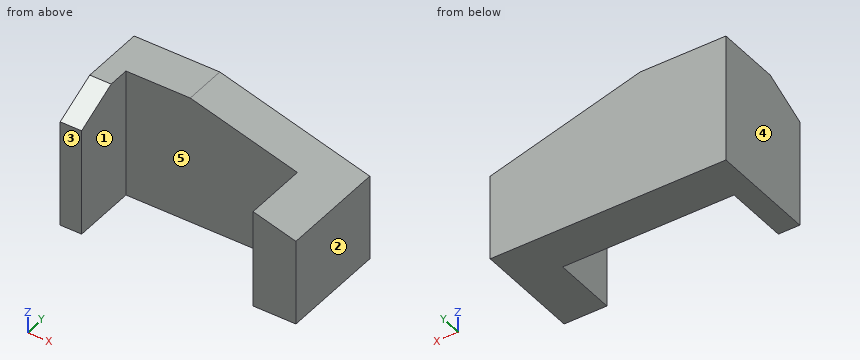
from build123d import *

# Parameters (mm, degrees)
F0_W     = 10
F0_H     = 20
F1_DEPTH = 60
F2_SIZE2 = 20
F2_SIZE  = 70
F3_SIZE2 = 20
F3_SIZE  = 10


with BuildPart() as f1:
    # F0 (on Top) → F1 (new body)
    with BuildSketch(Plane.XY):
        Polygon((40, 0), (0, 0), (0, -30), (10, -30), (10, -20), (40, -20), align=None)
        Polygon((110, 0), (40, 0), (40, -20), (90, -20), (90, -50), (110, -50), align=None)
        with Locations((5, -40)):
            Rectangle(F0_W, F0_H)
    extrude(amount=F1_DEPTH)

    # F2
    f2_edges = [f1.edges().sort_by_distance(p)[0] for p in [
        (110, -25, 60),
    ]]
    f2_side = f1.faces().sort_by_distance((58.870968, -17.258065, 60))[0]
    chamfer(f2_edges, length=F2_SIZE, length2=F2_SIZE2, reference=f2_side)

    # F3
    f3_edges = [f1.edges().sort_by_distance(p)[0] for p in [
        (5, -50, 60),
    ]]
    f3_side = f1.faces().sort_by_distance((5, -50, 30))[0]
    chamfer(f3_edges, length=F3_SIZE, length2=F3_SIZE2, reference=f3_side)


solid = f1.part
Check sheet for the modelled part. Datum: model origin and axes. Units: mm. Face numbers are marked on the shaded views. A direction names the side the tool comes from. Round coordinates to 2 decimals unless told otherwise and drop trailing zeros. Loops run counter-clockwise (first coordinate to the right, second up) from the corner with the lowest first, then second, coordinate; pieces in that order, holes last. Notation, with made-up numbers: (-32, -10) - (6, -10) arc R25 ccw to (6, 17) - close; hole circle Ø3 at (38, 31.25). An arc over 180 degrees is marked (long way). Answer as CSV lines item,"result". Start each with the question number.
Item 1: Section check A-A (y = -33). Record the boundary of the cut face in (x, z), and give its area (3 significant figures).
Item 2: Depth check by flat-ended pin: P1, Ø8, axis at x = 17.5, y = -37, coming from the -Z side; P2, Ø1.5, axis at x = 60.5, y = -20, coming from the +Z side. Enter the tip coordinate at first touch or a pass-through.
Item 3: Set-up check for the marked faces 1 and 2: record each of +Z, -Z, +X, -X, +Y, -Y from which the full face is reachable in a straight line by a thin tool's end or side.
Item 4: Section check D-D (y = -14). Record the boundary of the cut face in (x, z).
Item 5: Release check for a two-part mould opening along X. For the marked faces 3, 4 and 5 record: +X half, -X half, draft (parallel to the pull), parting line (faces both ways), or undercut.
Item 6: Scan lines: line 1 (X direction, y = -45.5, z = 11.5); line 2 (Y direction, x = 45.5, z = 16.5); line 3 (X direction, y = -22, z = 51.5). Record each from-to range of solid material in increasing order. Write a range as [from, to].
Item 7: Section check B-B (z = 5). Record the boundary of the cut face in (x, y), and give its area (3 significant figures).
Item 8: Section check C-C (y = -25). Record the boundary of the cut face in (x, z).
Report:
1,outline,"(0, 0) - (10, 0) - (10, 58.5) - (0, 58.5) - close; (90, 0) - (110, 0) - (110, 40) - (90, 45.71) - close"
1,area,"1,440 mm2"
2,P1,"passes through"
2,P2,"stops at z = 54.36"
3,face 1,"+Z, -Z, -Y"
3,face 2,"+Z, -Z, +X, +Y, -Y"
4,outline,"(0, 0) - (110, 0) - (110, 40) - (40, 60) - (0, 60) - close"
5,face 3,"draft"
5,face 4,"-X half"
5,face 5,"undercut"
6,line 1,"x = [0, 10], [90, 110]"
6,line 2,"y = [-20, 0]"
6,line 3,"x = [0, 10]"
7,outline,"(0, -50) - (10, -50) - (10, -20) - (90, -20) - (90, -50) - (110, -50) - (110, 0) - (0, 0) - close"
7,area,"3,100 mm2"
8,outline,"(0, 0) - (10, 0) - (10, 60) - (0, 60) - close; (90, 0) - (110, 0) - (110, 40) - (90, 45.71) - close"
